Verification items for the finished model (mm, model axes). A direction names the side the tool comes from. Coordinates: 2 decimals unless noted, no trailing zeros. Order: outer loops, then holes, each group sorted by start corner. A loop starts at its lowest first (then second) coordinate and runs counter-clockwise, first axis right, second up. Notation, with made-up numbers: M -14.5,-20.5 L 35.5,-20.5 A26 cw 35.5,-0.5 Z; hole C 77,31 d3. An arc over 180 degrees is marked long. Use one line per item in the form item = value. Start each with the question number.
```python
from build123d import *

# Parameters (mm, degrees)
SKETCH_W        = 100
SKETCH_H        = 100
PAD_DEPTH       = 10
SKETCH001_R     = 40
PAD001_DEPTH    = 30
SKETCH002_R     = 38
POCKET_DEPTH    = 55
SKETCH003_R     = 3
POCKET001_DEPTH = 10
SKETCH004_R     = 3
POCKET002_DEPTH = 10
SKETCH005_R     = 5
POCKET003_DEPTH = 5
FILLET_R        = 6


with BuildPart() as part:
    # Sketch → Pad (new body)
    with BuildSketch(Plane.XY):
        Rectangle(SKETCH_W, SKETCH_H)
    extrude(amount=PAD_DEPTH)

    # Sketch001 (on Face6 of Pad) → Pad001 (join)
    with BuildSketch(Plane.XY.offset(10)):
        Circle(SKETCH001_R)
    extrude(amount=PAD001_DEPTH)

    # Sketch002 (on Face8 of Pad001) → Pocket (cut)
    with BuildSketch(Plane.XY.offset(40)):
        Circle(SKETCH002_R)
    extrude(amount=-POCKET_DEPTH, mode=Mode.SUBTRACT)

    # Sketch003 (on Face4 of Pocket) → Pocket001 (cut)
    with BuildSketch(Plane(origin=(0, 0, 0), x_dir=(1, 0, 0), z_dir=(0, 0, -1))):
        with Locations((-36, 36)):
            Circle(SKETCH003_R)
        with Locations((36, 36)):
            Circle(SKETCH003_R)
        with Locations((36, -36)):
            Circle(SKETCH003_R)
        with Locations((-36, -36)):
            Circle(SKETCH003_R)
    extrude(amount=-POCKET001_DEPTH, mode=Mode.SUBTRACT)

    # Sketch004 (on Face4 of Pocket001) → Pocket002 (cut)
    with BuildSketch(Plane(origin=(0, 0, 0), x_dir=(1, 0, 0), z_dir=(0, 0, -1))):
        with Locations((-43, 43)):
            Circle(SKETCH004_R)
        with Locations((43, 43)):
            Circle(SKETCH004_R)
        with Locations((43, -43)):
            Circle(SKETCH004_R)
        with Locations((-43, -43)):
            Circle(SKETCH004_R)
    extrude(amount=-POCKET002_DEPTH, mode=Mode.SUBTRACT)

    # Sketch005 (on Face5 of Pocket002) → Pocket003 (cut)
    with BuildSketch(Plane.XY.offset(10)):
        with Locations((-36, 36)):
            Circle(SKETCH005_R)
        with Locations((36, 36)):
            Circle(SKETCH005_R)
        with Locations((36, -36)):
            Circle(SKETCH005_R)
        with Locations((-36, -36)):
            Circle(SKETCH005_R)
    extrude(amount=-POCKET003_DEPTH, mode=Mode.SUBTRACT)

    # Fillet
    fillet_edges = [part.edges().sort_by_distance(p)[0] for p in [
        (-50, -50, 5),
        (-50, 50, 5),
        (50, 50, 5),
        (50, -50, 5),
    ]]
    fillet(fillet_edges, radius=FILLET_R)


solid = part.part
```
1. Cross-section at C-C on x = 36. Enter the section's corners in (y, z), and give its area (3 significant figures).
2. Cross-section at D-D on z = 19. Enter the section's corners in (x, y).
3. Depth check by flat-ended pin: P1, Ø3, axis at x = 38, y = -37, coming from the +Z side; P2, Ø11, axis at x = 34.5, y = -34, coming from the +Z side; P3, Ø4, axis at x = 1, z = 34.5, coming from the +Y side. Enter the tip coordinate at first touch or a pass-through.
4. Material ranges on line 1 along Y through (x, z) = (0, 16); line 2 along Z through (x, y) = (-21, 45.5); line 3 along X through (y, z) = (-38.5, 3.5), recorded low to high.
5. Cross-section at A-A on y = 0. Enter the section's corners in (x, z), and give its area (3 significant figures).
6. Cross-section at B-B on x = 9.5. Enter the section's corners in (y, z), and give its area (3 significant figures).
7. Release check for a two-part mould opening along Y. For faces 1 (the flat face through (35.4, -14.6, 40)), 2 (the cylindrical face through (40.79, 40.97, 4.93)), 3 (the cylindrical face through (-48.289, 48.196, 5.07)) record: pulls with the +Y half, pulls with the -Y half, needs draft (parallel to the pull), parting line crosses it, or undercut.
8. Tool access check on faces 4 (the flat face through (50, -1, 5)), 5 (the cylindrical face through (32, 39, 8)). Record the directions out of +Z, -Z, +X, -X, +Y, -Y that give a thin tool (end or side, any length) a straight path to the whole face; none if there is none.
Final values:
q1.outline = M -50,0 L -39,0 L -39,5 L -41,5 L -41,10 L -50,10 Z; M -33,0 L -12.17,0 L -12.17,40 L -17.44,40 L -17.44,10 L -31,10 L -31,5 L -33,5 Z; M 12.17,0 L 33,0 L 33,5 L 31,5 L 31,10 L 17.44,10 L 17.44,40 L 12.17,40 Z; M 39,0 L 50,0 L 50,10 L 41,10 L 41,5 L 39,5 Z
q1.area = 913 mm2
q2.outline = C 0,0 d80; hole C 0,0 d76
q3.P1 = 5
q3.P2 = 10
q3.P3 = 40
q4.line_1 = -40 to -38, 38 to 40
q4.line_2 = 0 to 10
q4.line_3 = -50 to -37.66, -34.34 to 34.34, 37.66 to 50
q5.outline = M -50,0 L -38,0 L -38,40 L -40,40 L -40,10 L -50,10 Z; M 38,0 L 50,0 L 50,10 L 40,10 L 40,40 L 38,40 Z
q5.area = 360 mm2
q6.outline = M -50,0 L -36.79,0 L -36.79,40 L -38.86,40 L -38.86,10 L -50,10 Z; M 36.79,0 L 50,0 L 50,10 L 38.86,10 L 38.86,40 L 36.79,40 Z
q6.area = 388 mm2
q7.face_1 = needs draft
q7.face_2 = undercut
q7.face_3 = pulls with the +Y half
q8.face_4 = +Z, -Z, +X, +Y, -Y
q8.face_5 = +Z
